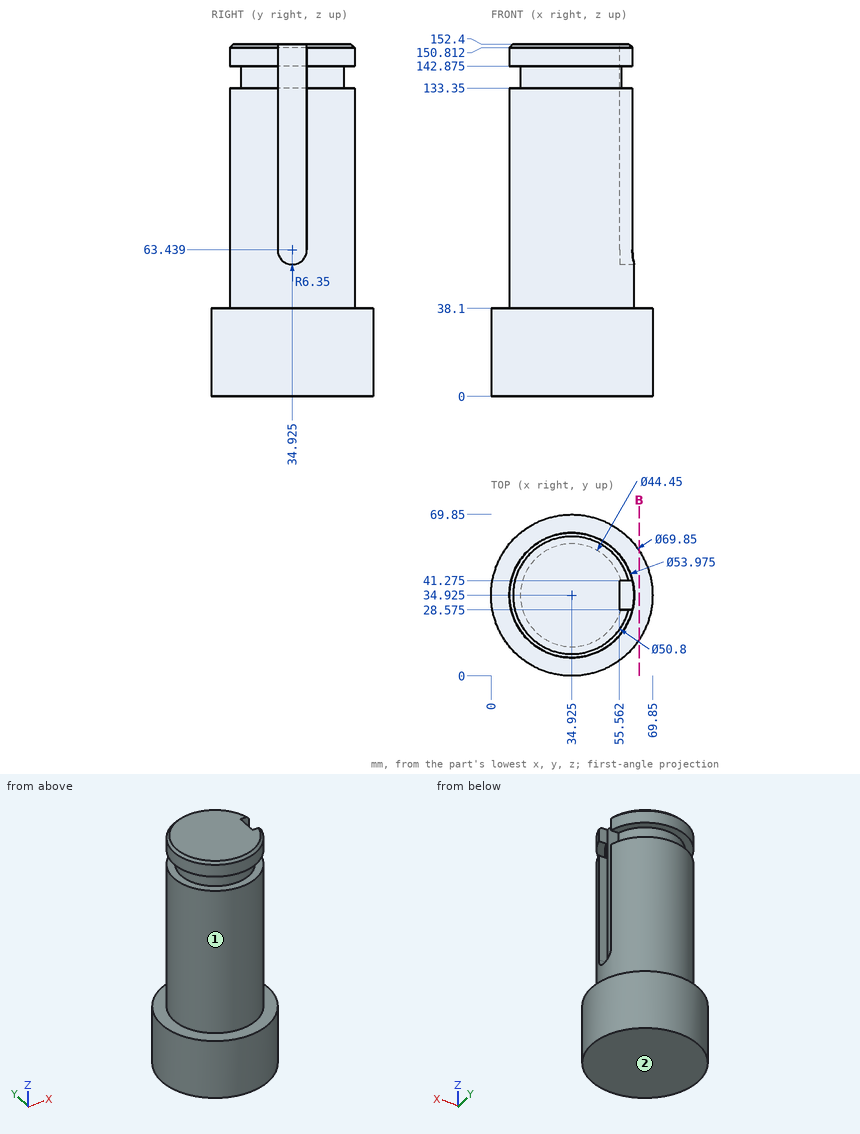
Geometry check sheet. Reference: drawing and pictorial views, mm from the part's lowest x, y, z. A direction names the side the tool comes from. Give positions to 0.01 mm unless a question says otherwise; leave off trailing zeros. Write each loop counter-clockwise with the first axis right and the second up, starting at its lowest first coordinate (ties: lowest second). Pieces come first, ordered by that corner, then holes. Notation, with made-up numbers: M 23.5,-25 L 62.5,-25 A20 ccw 62.5,-5 Z; hole C -39.75,-30.5 d9. An arc over 180 degrees is marked long. Put each result on its own line as item: value. Start each with the question number.
1. Go/stop test with flat-tipped pins: pin 1 Ø1.5 at (y, z) = (12, 113) entering from -X (1 decimal); pin 2 Ø1.5 at (x, z) = (34.5, 29.5) entering from +Y; pin 3 Ø1.7 at (x, z) = (59.5, 129) entering from +Y (1 decimal); pin 4 Ø16 at (x, y) = (39.5, 37) entering from -Z. Record where each tip stops, or that it passes through.
2. Scan lines: line 1 along X through (y, z) = (32, 134.5); line 2 along Y through (x, z) = (44.5, 129); line 3 along Y through (x, z) = (45.5, 85) (1 decimal). Record each from-to range of solid material in increasing order. Write a range as [from, to].
3. Set-up check for the marked faces 1 and 2: record each of +Z, -Z, +X, -X, +Y, -Y from which the full face is reachable in a straight line by a thin tool's end or side.
4. Section check B-B (x = 64). Record the cut outline in (y, z) (1 decimal).
Answer list:
1. pin 1: x = 19.5
1. pin 2: y = 69.85
1. pin 3: y = 47.8
1. pin 4: z = 0
2. line 1: [12.89, 55.56]
2. line 2: [9.69, 60.16]
2. line 3: [10.1, 59.8]
3. face 1: +Z
3. face 2: -Z, +X, -X, +Y, -Y
4. outline: M 15.6,0 L 54.3,0 L 54.3,38.1 L 15.6,38.1 Z
